Can you work these out from the model? Positions are in its coordinate system, mm. A direction names the side the tool comes from. Round coordinates to 2 decimals unless told otherwise and drop trailing zeros. Loops run counter-clockwise (first coordinate to the right, second up) from the corner with the lowest first, then second, coordinate; pieces in that order, holes last. Notation, with made-up numbers: (30.5, 12) -> (85.5, 12) arc R14 ccw to (85.5, 20) -> close; hole circle Ø7 at (30, -5). An arc over 180 degrees is marked (long way). Answer as a JSON object with one key per item and string values.
```python
from build123d import *

# Parameters (mm, degrees)
SKETCH1_W           = 50
SKETCH1_H           = 25
BOSS_EXTRUDE1_DEPTH = 25
BOSS_EXTRUDE2_DEPTH = 25
SKETCH4_R           = 6.625
CUT_EXTRUDE1_DEPTH  = 50
SKETCH5_R           = 3.1
CUT_EXTRUDE2_DEPTH  = 90.697578477
SKETCH6_R           = 3.125
CUT_EXTRUDE3_DEPTH  = 112.338788217


with BuildPart() as part:
    # Sketch1 → Boss-Extrude1 (new body)
    with BuildSketch(Plane.XY):
        Rectangle(SKETCH1_W, SKETCH1_H)
    extrude(amount=BOSS_EXTRUDE1_DEPTH)

    # Sketch3 → Boss-Extrude2 (add)
    with BuildSketch(Plane.XY.offset(25)):
        Polygon((-25, 12.5), (-74.513403437, 19.458655048), (-71.173249014, 43.225088698), (-21.659845577, 36.26643365), (21.659845577, 36.26643365), (71.173249014, 43.225088698), (74.513403437, 19.458655048), (25, 12.5), align=None)
    extrude(amount=-BOSS_EXTRUDE2_DEPTH)

    # Sketch4 → Cut-Extrude1 (cut)
    with BuildSketch(Plane(origin=(-75.75190811, 10.646236396, 0), x_dir=(0, 0, 1), z_dir=(-0.9902680687415705, 0.13917310096006502, 0))):
        with Locations(Location((12.5, 20.899023335, 0), (0, 0, 270))):
            Circle(SKETCH4_R)
    cut_extrude1 = extrude(amount=-CUT_EXTRUDE1_DEPTH, mode=Mode.SUBTRACT)

    # Mirror1: Cut-Extrude1 across plane
    add(cut_extrude1.mirror(Plane(origin=(0, 0, 0), x_dir=(0, 0, 1), z_dir=(1, 0, 0))), mode=Mode.SUBTRACT)

    # Sketch5 → Cut-Extrude2 (cut, through all)
    with BuildSketch(Plane.XY.offset(25)):
        with Locations((-62.940645538, 29.950140863)):
            Circle(SKETCH5_R)
        with Locations((-38.18394382, 26.470813339)):
            Circle(SKETCH5_R)
        with Locations((38.18394382, 26.470813339)):
            Circle(SKETCH5_R)
        with Locations((62.940645538, 29.950140863)):
            Circle(SKETCH5_R)
    extrude(amount=-CUT_EXTRUDE2_DEPTH, mode=Mode.SUBTRACT)

    # Sketch6 → Cut-Extrude3 (cut, through all)
    with BuildSketch(Plane(origin=(25, 0, 0), x_dir=(0, 0, -1), z_dir=(1, 0, 0))):
        with Locations((-20, 7.5)):
            Circle(SKETCH6_R)
        with Locations((-5, 7.5)):
            Circle(SKETCH6_R)
        with Locations((-5, -7.5)):
            Circle(SKETCH6_R)
        with Locations((-20, -7.5)):
            Circle(SKETCH6_R)
    extrude(amount=-CUT_EXTRUDE3_DEPTH, mode=Mode.SUBTRACT)


solid = part.part
```
Q1. On a 3-axis mill with a long thin cutter (end or side, diameter ignored), from which of +Z, -Z, +X, -X, +Y, -Y can I reach the whole of each face in a straight line? I mean faces 1 (the flat face through (25, 0, 12)), 2 (the flat face through (-23.317, 24.475, 12.593)), 3 (the flat face through (46.1, 39.7, 12.7)). Say none if no direction works.
Determined:
{"face 1": "+Z, -Z, +X, -Y", "face 2": "none", "face 3": "+Z, -Z, +Y"}
Q2. We'd pull the mould along Y, two halves only. Please class faces 4 (the flat face through (-25, 0, 12)), 5 (the flat face through (50.103, 16.028, 12.675)), 6 (the cylindrical face through (-60.08, 28.76, 3.37)), 7 (the flat face through (-72.124, 36.457, 7.119)): pulls with the +Y half, pulls with the -Y half, needs draft (parallel to the pull), parting line crosses it, or undercut.
Determined:
{"face 4": "needs draft", "face 5": "pulls with the -Y half", "face 6": "undercut", "face 7": "pulls with the +Y half"}
Q3. I'm going to push flat-ended pins straight in: pin 1 (4 mm diameter, centred on x = 26.5, z = 8, fed in from -Y); pin 2 (1 mm diameter, centred on y = 36.5, z = 22, fed in from +X); pin 3 (7.5 mm diameter, centred on x = 10, z = 16, fed in from +Y); pin 4 (6 mm diameter, centred on x = 53, z = 3, fed in from +Y). Where does each tip first touch, or does it pass through?
Determined:
{"pin 1": "y = -12.5", "pin 2": "x = 72.19", "pin 3": "y = 36.27", "pin 4": "y = 41.09"}
Q4. I want a section at B-B, the plane y = -7.5. Write out the boundary of the cut face in (x, z) (3 decimals).
Determined:
{"outline": "(-25, 0) -> (25, 0) -> (25, 1.875) -> (-25, 1.875) -> close; (-25, 8.125) -> (25, 8.125) -> (25, 16.875) -> (-25, 16.875) -> close; (-25, 23.125) -> (25, 23.125) -> (25, 25) -> (-25, 25) -> close"}
Q5. If I drill on L1, parallel to Y at x = 7, z = 5 (3 decimals); L2, parallel to X at y = 27.5, z = 1.5; L3, parallel to Z at x = 2, y = -8.5, over which ranges is the centre line in solid material (lowest first)? Write a range as [from, to].
Determined:
{"L1": "[-12.5, -10.625], [-4.375, 4.375], [10.625, 36.266]", "L2": "[-73.38, -64.84], [-61.04, -41.11], [-35.26, 35.26], [41.11, 61.04], [64.84, 73.38]", "L3": "[0, 2.04], [7.96, 17.04], [22.96, 25]"}
Q6. I want a section at A-A, the plane z = 3.75. Write out the boundary of the cut face in (x, y), then the cut area to 3 significant figures.
Determined:
{"outline": "(-74.51, 19.46) -> (-25, 12.5) -> (-25, 10.36) -> (25, 10.36) -> (25, 12.5) -> (74.51, 19.46) -> (71.17, 43.23) -> (21.66, 36.27) -> (-21.66, 36.27) -> (-71.17, 43.23) -> close; (-25, -12.5) -> (25, -12.5) -> (25, -10.36) -> (-25, -10.36) -> close; (-25, -4.64) -> (25, -4.64) -> (25, 4.64) -> (-25, 4.64) -> close; hole circle Ø6.2 at (-62.94, 29.95); hole circle Ø6.2 at (-38.18, 26.47); hole circle Ø6.2 at (38.18, 26.47); hole circle Ø6.2 at (62.94, 29.95)", "area": "4,070 mm²"}
Q7. I want a section at D-D, the plane z = 15. Write out the boundary of the cut face in (x, y).
Determined:
{"outline": "(-74.51, 19.46) -> (-25, 12.5) -> (-25, -12.5) -> (25, -12.5) -> (25, 12.5) -> (74.51, 19.46) -> (73.7, 25.27) -> (24.18, 18.31) -> (22.48, 30.46) -> (71.99, 37.42) -> (71.17, 43.23) -> (21.66, 36.27) -> (-21.66, 36.27) -> (-71.17, 43.23) -> (-71.99, 37.42) -> (-22.48, 30.46) -> (-24.18, 18.31) -> (-73.7, 25.27) -> close"}
Q8. I want a section at C-C, the plane x = 3. Write out the boundary of the cut face in (y, z) (3 decimals).
Determined:
{"outline": "(-12.5, 0) -> (36.266, 0) -> (36.266, 25) -> (-12.5, 25) -> close; hole circle Ø6.25 at (-7.5, 5); hole circle Ø6.25 at (-7.5, 20); hole circle Ø6.25 at (7.5, 5); hole circle Ø6.25 at (7.5, 20)"}
